Geometry check sheet. Reference: the model listing, model coordinates, mm. A direction names the side the tool comes from. Give positions to 0.01 mm unless a question says otherwise; leave off trailing zeros. Write each loop counter-clockwise with the first axis right and the second up, starting at its lowest first coordinate (ties: lowest second). Pieces come first, ordered by that corner, then holes.
(1) Cross-section at B-B (x = 5). Record the boundary of the cut face in (y, z).
(2) Cross-section at D-D (x = 20). Record the boundary of the cut face in (y, z), and give its area (3 significant figures).
(3) Thickness scan on line 1 along X through (y, z) = (31, 2); line 2 along Z through (x, y) = (9, 4); line 3 along X through (y, z) = (-26, -30.5). Record the ranges inside material, lowest first.
(4) Depth check by flat-ended pin: P1, Ø3.5, axis at x = 29, y = 31.5, coming from the +Z side; P2, Ø8, axis at x = 3.5, y = 30.5, coming from the -Z side; P3, Ø10.5, axis at y = -10.5, z = -21.5, coming from the -X side; P4, Ø8, axis at x = 19, z = -27, coming from the +Y side. Enter the tip coordinate at first touch or a pass-through.
(5) Cross-section at C-C (z = -37). Record the boundary of the cut face in (x, y), and give its area (3 significant figures).
(6) Mould release check, pull along Y, two halves, no side actions. Record for faces 1 (the cylindrical face through (0.562, 41.748, 3.091)), 2 (the cylindrical face through (25.62, -10.35, -28.5)), 3 (the flat face through (29, -10, -21)): +Y half, -Y half, draft (parallel to the pull), parting line (faces both ways), or undercut.
(7) Cross-section at A-A (y = 6). Record the boundary of the cut face in (x, z), and give its area (3 significant figures).
(8) Tool access check on faces 4 (the cylindrical face through (36.465, 38.115, -38.216)), 5 (the flat face through (26, -3.5, -12)), 6 (the cylindrical face through (5.46, 15.02, 2.07)), 7 (the cylindrical face through (24.37, -18.1, -0.57)), 8 (the cylindrical face through (36.53, -13.03, -18.21)). Record the directions out of +Z, -Z, +X, -X, +Y, -Y that give a thin tool (end or side, any length) a straight path to the whole face; none if there is none.
```python
from build123d import *

# Parameters (mm, degrees)
SKETCH1_W           = 34
SKETCH1_H           = 43
SKETCH1_R           = 2.15
BOSS_EXTRUDE2_DEPTH = 5
SKETCH2_W           = 5
SKETCH2_H           = 43
BOSS_EXTRUDE3_DEPTH = 53
SKETCH3_R           = 3.55
SKETCH3_R_2         = 2.15
CUT_EXTRUDE1_DEPTH  = 4.2
SKETCH5_R           = 1.65
SKETCH5_R_2         = 11.2
CUT_EXTRUDE2_DEPTH  = 5
FILLET1_R           = 3
BOSS_EXTRUDE6_DEPTH = 30
SKETCH9_R           = 4.15
CUT_EXTRUDE3_DEPTH  = 10
BOSS_EXTRUDE9_DEPTH = 17
SKETCH11_R          = 4
CUT_EXTRUDE4_DEPTH  = 5
FILLET5_R           = 2
FILLET6_R           = 2
FILLET7_R           = 2


with BuildPart() as part:
    # Sketch1 → Boss-Extrude2 (new body)
    with BuildSketch(Plane.XY):
        with Locations((17, 21.5)):
            Rectangle(SKETCH1_W, SKETCH1_H)
        with Locations((5, 31.5)):
            Circle(SKETCH1_R, mode=Mode.SUBTRACT)
        with Locations((29, 31.5)):
            Circle(SKETCH1_R, mode=Mode.SUBTRACT)
        with Locations((5, 11.5)):
            Circle(SKETCH1_R, mode=Mode.SUBTRACT)
        with Locations((29, 11.5)):
            Circle(SKETCH1_R, mode=Mode.SUBTRACT)
    extrude(amount=BOSS_EXTRUDE2_DEPTH)

    # Sketch2 → Boss-Extrude3 (add)
    with BuildSketch(Plane.XY.offset(5)):
        with Locations((36.5, 21.5)):
            Rectangle(SKETCH2_W, SKETCH2_H)
    extrude(amount=-BOSS_EXTRUDE3_DEPTH)

    # Sketch3 → Cut-Extrude1 (cut)
    with BuildSketch(Plane(origin=(0, 0, 0), x_dir=(-1, 0, 0), z_dir=(0, 0, -1))):
        with Locations((-29, 31.5)):
            Circle(SKETCH3_R)
        with Locations((-29, 31.5)):
            Circle(SKETCH3_R_2, mode=Mode.SUBTRACT)
        with Locations((-5, 31.5)):
            Circle(SKETCH3_R)
        with Locations((-5, 31.5)):
            Circle(SKETCH3_R_2, mode=Mode.SUBTRACT)
        with Locations((-5, 11.5)):
            Circle(SKETCH3_R)
        with Locations((-5, 11.5)):
            Circle(SKETCH3_R_2, mode=Mode.SUBTRACT)
        with Locations((-29, 11.5)):
            Circle(SKETCH3_R)
        with Locations((-29, 11.5)):
            Circle(SKETCH3_R_2, mode=Mode.SUBTRACT)
    extrude(amount=-CUT_EXTRUDE1_DEPTH, mode=Mode.SUBTRACT)

    # Sketch5 → Cut-Extrude2 (cut)
    with BuildSketch(Plane.ZY.offset(-34)):
        with Locations((-6, 6)):
            Circle(SKETCH5_R)
        with Locations((-37, 6)):
            Circle(SKETCH5_R)
        with Locations((-37, 37)):
            Circle(SKETCH5_R)
        with Locations((-21.5, 21.5)):
            Circle(SKETCH5_R_2)
        with Locations((-6, 37)):
            Circle(SKETCH5_R)
    extrude(amount=-CUT_EXTRUDE2_DEPTH, mode=Mode.SUBTRACT)

    # Fillet1
    fillet1_edges = [part.edges().sort_by_distance(p)[0] for p in [
        (36.5, 43, -48),
        (17, 43, 0),
        (0, 43, 2.5),
    ]]
    fillet(fillet1_edges, radius=FILLET1_R)

    # Sketch7 → Boss-Extrude6 (add)
    with BuildSketch(Plane.XZ):
        Polygon((0, 5), (39, 5), (39, 0), (39, -48), (34, -48), (34, 0), (0, 0), align=None)
    extrude(amount=BOSS_EXTRUDE6_DEPTH)

    # Sketch9 → Cut-Extrude3 (cut)
    with BuildSketch(Plane(origin=(39, 0, 0), x_dir=(0, 0, -1), z_dir=(1, 0, 0))):
        with Locations((21.5, -10.5)):
            Circle(SKETCH9_R)
    extrude(amount=-CUT_EXTRUDE3_DEPTH, mode=Mode.SUBTRACT)

    # Sketch10 → Boss-Extrude9 (add)
    with BuildSketch(Plane.ZY.offset(-34)):
        with BuildLine():
            Line((0, -3.5), (-21.5, -3.5))
            ThreePointArc((-21.5, -3.5), (-28.5, -10.5), (-21.5, -17.5))
            Line((-21.5, -17.5), (0, -17.5))
            Line((0, -17.5), (0, -3.5))
        make_face()
    extrude(amount=BOSS_EXTRUDE9_DEPTH)

    # Sketch11 → Cut-Extrude4 (cut)
    with BuildSketch(Plane(origin=(34, 0, 0), x_dir=(0, 0, -1), z_dir=(1, 0, 0))):
        with Locations((21.5, -10.5)):
            Circle(SKETCH11_R)
    extrude(amount=-CUT_EXTRUDE4_DEPTH, mode=Mode.SUBTRACT)

    # Fillet5
    fillet5_edges = [part.edges().sort_by_distance(p)[0] for p in [
        (17, -30, 0),
        (36.5, -30, -48),
    ]]
    fillet(fillet5_edges, radius=FILLET5_R)

    # Fillet6
    fillet6_edges = [part.edges().sort_by_distance(p)[0] for p in [
        (25.5, -3.5, 0),
        (25.5, -17.5, 0),
        (17, -10.5, 0),
    ]]
    fillet(fillet6_edges, radius=FILLET6_R)

    # Fillet7
    fillet7_edges = [part.edges().sort_by_distance(p)[0] for p in [
        (39, -30, -20.5),
        (39, -29.414213562, -47.414213562),
        (39, 43, -20),
        (39, 42.121320344, -47.121320344),
        (34, 43, -21),
        (34, 42.121320344, -47.121320344),
        (34, -30, -23),
        (34, -29.414213562, -47.414213562),
        (39, 6, -48),
        (34, 6, -48),
    ]]
    fillet(fillet7_edges, radius=FILLET7_R)


solid = part.part
```
Reply:
1. outline: (-30, 2) arc R2 ccw to (-28, 0) - (7.95, 0) - (7.95, 4.2) - (9.35, 4.2) - (9.35, 5) - (-30, 5) - close; (13.65, 4.2) - (15.05, 4.2) - (15.05, 0) - (27.95, 0) - (27.95, 4.2) - (29.35, 4.2) - (29.35, 5) - (13.65, 5) - close; (33.65, 4.2) - (35.05, 4.2) - (35.05, 0) - (40, 0) arc R3 ccw to (43, 3) - (43, 5) - (33.65, 5) - close
2. outline: (-30, 2) arc R2 ccw to (-28, 0) - (-19.5, 0) arc R2 cw to (-17.5, -2) - (-17.5, -21.5) arc R7 ccw to (-3.5, -21.5) - (-3.5, -2) arc R2 cw to (-1.5, 0) - (40, 0) arc R3 ccw to (43, 3) - (43, 5) - (-30, 5) - close
2. area: 742 mm2
3. line 1: x = 0 to 1.49, 8.51 to 25.49, 32.51 to 39
3. line 2: z = 0 to 5
3. line 3: x = 34 to 39
4. P1: passes through
4. P2: stops at z = 0
4. P3: stops at x = 17
4. P4: stops at y = -3.66
5. outline: (34, -28) arc R2 ccw to (36, -30) - (37, -30) arc R2 ccw to (39, -28) - (39, 4.35) - (34, 4.35) - close; (34, 7.65) - (39, 7.65) - (39, 35.35) - (34, 35.35) - close; (34, 38.65) - (39, 38.65) - (39, 41) arc R2 ccw to (37, 43) - (36, 43) arc R2 ccw to (34, 41) - close
5. area: 329 mm2
6. face 1: +Y half
6. face 2: parting line
6. face 3: undercut
7. outline: (0, 0) - (34, 0) - (34, -4.35) - (39, -4.35) - (39, 5) - (0, 5) - close; (34, -46) arc R2 ccw to (36, -48) - (37, -48) arc R2 ccw to (39, -46) - (39, -38.65) - (34, -38.65) - close; (34, -35.35) - (39, -35.35) - (39, -7.65) - (34, -7.65) - close
7. area: 400 mm2
8. face 4: +X, -X
8. face 5: -Z, -X, +Y
8. face 6: -Z
8. face 7: -Z, -X, -Y
8. face 8: +X
